Geometry: final body of the model. Coordinates: model frame, mm. Face numbers are marked on the shaded views. A direction names the side the tool comes from. Give positions to 0.01 mm unless a question says otherwise; leave off trailing zeros. Loops run counter-clockwise (first coordinate to the right, second up) from the corner with the lowest first, then second, coordinate; pieces in that order, holes last.
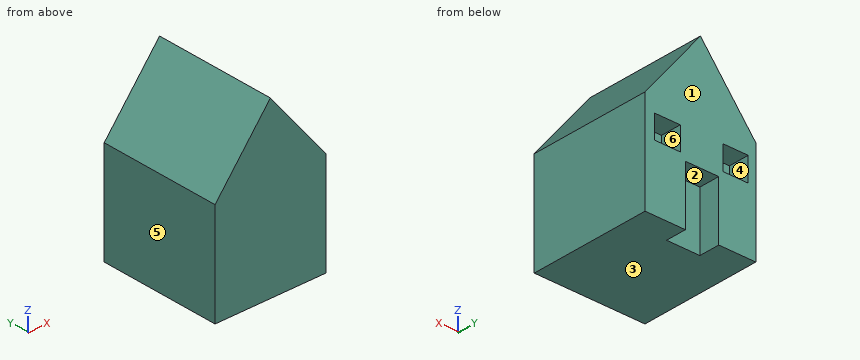
from build123d import *

# Parameters (mm, degrees)
F0_W     = 92.0496
F0_H     = 85.240435
F2_DEPTH = 101.6
F1_W     = 21.440845
F1_H     = 19.349056
F1_W_2   = 20.917898
F1_H_2   = 19.872003
F1_W_3   = 27.716208
F1_H_3   = 48.895583
F3_DEPTH = 17.272


with BuildPart() as f2:
    # F0 (on Front) → F2 (new body)
    with BuildSketch(Plane.XZ):
        Polygon((1.30194, 94.392009), (-44.72286, 36.344852), (47.32674, 36.344852), align=None)
        with Locations((1.30194, -6.275365)):
            Rectangle(F0_W, F0_H)
    extrude(amount=F2_DEPTH)

    # F1 (on Front) → F3 (cut)
    with BuildSketch(Plane.XZ):
        with Locations((28.762107, 14.642532)):
            Rectangle(F1_W, F1_H)
        with Locations((-27.977687, 14.904006)):
            Rectangle(F1_W_2, F1_H_2)
        with Locations((-0.075163, -24.447791)):
            Rectangle(F1_W_3, F1_H_3)
    extrude(amount=F3_DEPTH, mode=Mode.SUBTRACT)


solid = f2.part
Item 1: Ray query, probe 1 along X at (y, z) = (-15, 21.5); probe 2 along Z at (x, y) = (35, -8); probe 3 along Y at (x, z) = (-4, -4.5). Return the intervals inside material, ascending.
Values follow:
probe 1: x = -44.72 to -38.44, -17.52 to 18.04, 39.48 to 47.33
probe 2: z = -48.9 to 4.97, 24.32 to 51.89
probe 3: y = -101.6 to -17.27
Item 2: Section query D-D on y = -43. Return loops of the section in (x, z).
Values follow:
outline: (-44.72, -48.9) - (47.33, -48.9) - (47.33, 36.34) - (1.3, 94.39) - (-44.72, 36.34) - close
Item 3: Section query C-C on x = -25. Return loops of the section in (y, z).
Values follow:
outline: (-101.6, -48.9) - (0, -48.9) - (0, 4.97) - (-17.27, 4.97) - (-17.27, 24.84) - (0, 24.84) - (0, 61.22) - (-101.6, 61.22) - close
Item 4: Section query B-B on z = 21. Return loops of the section in (x, y), plus the area to 3 significant figures.
Values follow:
outline: (-44.72, -101.6) - (47.33, -101.6) - (47.33, 0) - (39.48, 0) - (39.48, -17.27) - (18.04, -17.27) - (18.04, 0) - (-17.52, 0) - (-17.52, -17.27) - (-38.44, -17.27) - (-38.44, 0) - (-44.72, 0) - close
area: 8,620 mm2
Item 5: Section query A-A on y = -13.5. Return loops of the section in (x, z), plus the area to 3 significant figures.
Values follow:
outline: (-44.72, -48.9) - (-13.93, -48.9) - (-13.93, 0) - (13.78, 0) - (13.78, -48.9) - (47.33, -48.9) - (47.33, 36.34) - (1.3, 94.39) - (-44.72, 36.34) - close; hole (-38.44, 4.97) - (-17.52, 4.97) - (-17.52, 24.84) - (-38.44, 24.84) - close; hole (18.04, 4.97) - (39.48, 4.97) - (39.48, 24.32) - (18.04, 24.32) - close
area: 8,330 mm2
Item 6: Pin query (flat end, axial travel): pin 1 (6 mm diameter, centred on x = 30.5, z = -2.5, fed in from +Y); pin 2 (10 mm diameter, centred on x = -22.5, y = -31, fed in from +Z); pin 3 (8 mm diameter, centred on y = -23.5, z = 43, fed in from +X); pin 4 (14 mm diameter, centred on x = 32.5, y = -6, fed in from +Z). Return the tip coordinate at first contact, or that it passes through.
Values follow:
pin 1: stops at y = 0
pin 2: stops at z = 70.68
pin 3: stops at x = 45.22
pin 4: stops at z = 63.87
Item 7: Set-up query: the marked faces 1 and 2. Return all of +Z, -Z, +X, -X, +Y, -Y with unobstructed straight access to the full face (end or side cutting, diameter ignored); none if empty.
Values follow:
face 1: +Z, -Z, +X, -X, +Y
face 2: -Z, +Y
Item 8: Draft query along Z for the marked faces 3, 4, 5 and 6. Return one class per face: +Z half, -Z half, draft (parallel to the pull), parting line (faces both ways), or undercut.
Values follow:
face 3: -Z half
face 4: undercut
face 5: draft
face 6: undercut
